The figure shows three views and two pictorial views of one solid part (mm, origin at its lowest corner). Answer the questions. A direction names the side the tool comes from. Round coordinates to 2 decimals unless told otherwise and drop trailing zeros. Loops run counter-clockwise (first coordinate to the right, second up) from the corner with the lowest first, then second, coordinate; pieces in that order, holes last. Notation, with made-up numbers: (32, 55.5) -> (87, 55.5) arc R37 ccw to (87, 91.5) -> close; hole circle Ø8 at (-31.5, -4). An arc over 180 degrees is marked (long way). Write each question's results on one line, items separated by ' | '. Start each with the question number.
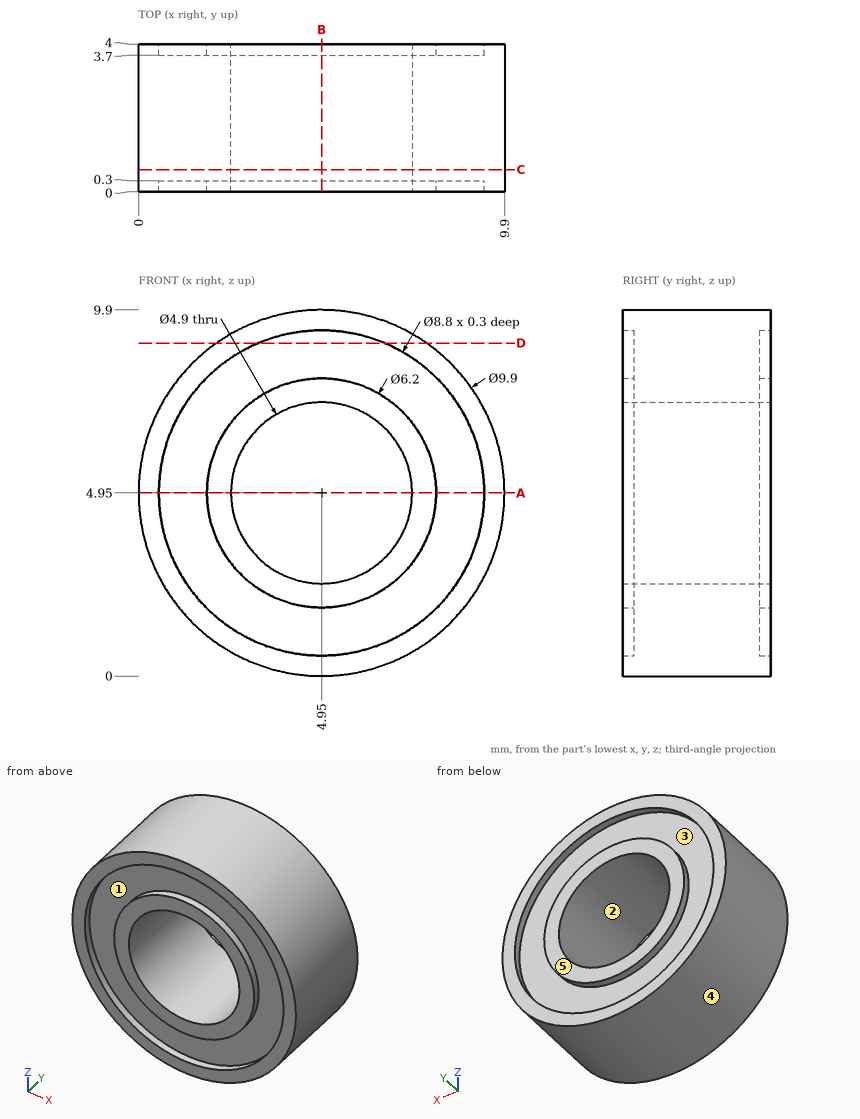
Item 1: Determine the mould class of the marked faces 3, 4 and 5 for opening direction Z: +Z half, -Z half, draft (parallel to the pull), parting line (faces both ways), or undercut.
Item 2: The part is cut by section B-B, the plane x = 4.95. Give the vertices of the cut face in (y, z), plus the area to 3 significant figures.
Item 3: The part is cut by section C-C, the plane y = 0.6. Give the vertices of the cut face in (x, z), plus the area to 3 significant figures.
Item 4: The part is cut by section D-D, the plane z = 9. Give the vertices of the cut face in (x, y).
Item 5: For the marked faces 1 and 2, determine the directions among +Z, -Z, +X, -X, +Y, -Y from which every point of the face is accessible in a straight line to the end or side of a thin tool.
Item 6: The part is cut by section A-A, the plane z = 4.95. Give the vertices of the cut face in (x, y).
Item 7: Straight lines are drawn through the part: L1, parallel to Z at x = 4.95, y = 3.85; L2, parallel to Z at x = 4.95, y = 1.8; L3, parallel to X at y = 3.2, z = 9.25. For each, find the intervals that lie inside material, in ascending order. Write a range as [from, to].
Item 8: Each of these flat-tipped pins is pushed along its axis until it touches: pin 1 Ø2 at (x, y) = (1.5, 2) entering from +Z; pin 2 Ø1 at (y, z) = (2.5, 7.5) entering from -X; pin 3 Ø1.5 at (x, y) = (8, 1) entering from -Z. Where does it stop, or does it pass through?
Report:
1) face 3: undercut | face 4: parting line | face 5: draft
2) outline: (0, 0) -> (4, 0) -> (4, 0.55) -> (3.7, 0.55) -> (3.7, 1.85) -> (4, 1.85) -> (4, 2.5) -> (0, 2.5) -> (0, 1.85) -> (0.3, 1.85) -> (0.3, 0.55) -> (0, 0.55) -> close; (0, 7.4) -> (4, 7.4) -> (4, 8.05) -> (3.7, 8.05) -> (3.7, 9.35) -> (4, 9.35) -> (4, 9.9) -> (0, 9.9) -> (0, 9.35) -> (0.3, 9.35) -> (0.3, 8.05) -> (0, 8.05) -> close | area: 18.4 mm2
3) outline: circle Ø9.9 at (4.95, 4.95); hole circle Ø4.9 at (4.95, 4.95) | area: 58.1 mm2
4) outline: (2.1, 0) -> (3.23, 0) -> (3.23, 0.3) -> (6.67, 0.3) -> (6.67, 0) -> (7.8, 0) -> (7.8, 4) -> (6.67, 4) -> (6.67, 3.7) -> (3.23, 3.7) -> (3.23, 4) -> (2.1, 4) -> close
5) face 1: -Y | face 2: +Y, -Y
6) outline: (0, 0) -> (0.55, 0) -> (0.55, 0.3) -> (1.85, 0.3) -> (1.85, 0) -> (2.5, 0) -> (2.5, 4) -> (1.85, 4) -> (1.85, 3.7) -> (0.55, 3.7) -> (0.55, 4) -> (0, 4) -> close; (7.4, 0) -> (8.05, 0) -> (8.05, 0.3) -> (9.35, 0.3) -> (9.35, 0) -> (9.9, 0) -> (9.9, 4) -> (9.35, 4) -> (9.35, 3.7) -> (8.05, 3.7) -> (8.05, 4) -> (7.4, 4) -> close
7) L1: z = [0, 0.55], [1.85, 2.5], [7.4, 8.05], [9.35, 9.9] | L2: z = [0, 2.5], [7.4, 9.9] | L3: x = [2.5, 7.4]
8) pin 1: stops at z = 9.25 | pin 2: stops at x = 0.44 | pin 3: stops at z = 0.57
